```python
from build123d import *

# Parameters (mm, degrees)
EXTRUDE_1_DEPTH     = 3
SKETCH_2_R          = 2
SKETCH_2_W          = 80
SKETCH_2_H          = 35.5
CUT_EXTRUDE_1_DEPTH = 10
SKETCH_5_R          = 3
CUT_EXTRUDE_4_DEPTH = 234.518735865
FILLET_1_R          = 10
FILLET_2_R          = 3
FILLET_3_R          = 2


with BuildPart() as part:
    # 草图1 → 凸台-拉伸1 (new body)
    with BuildSketch(Plane(origin=(0, 0, 0), x_dir=(1, 0, 0), z_dir=(0, 1, 0))):
        with BuildLine():
            Line((-55, 0), (55, 0))
            Line((55, 0), (55, 35.5))
            Line((55, 35.5), (147.5, 35.5))
            Line((147.5, 35.5), (147.5, 66))
            Line((147.5, 66), (204, 66))
            Line((204, 66), (204, 26))
            Line((204, 26), (219, 26))
            Line((219, 26), (219, 73))
            ThreePointArc((219, 73), (216.656854249, 78.656854249), (211, 81))
            Line((211, 81), (132.5, 81))
            Line((132.5, 81), (132.5, 50.5))
            Line((132.5, 50.5), (-132.5, 50.5))
            Line((-132.5, 50.5), (-132.5, 81))
            Line((-132.5, 81), (-211, 81))
            ThreePointArc((-211, 81), (-216.656854249, 78.656854249), (-219, 73))
            Line((-219, 73), (-219, 26))
            Line((-219, 26), (-204, 26))
            Line((-204, 26), (-204, 66))
            Line((-204, 66), (-147.5, 66))
            Line((-147.5, 66), (-147.5, 35.5))
            Line((-147.5, 35.5), (-55, 35.5))
            Line((-55, 35.5), (-55, 0))
        make_face()
    extrude(amount=EXTRUDE_1_DEPTH)

    # 草图2 → 切除-拉伸1 (cut)
    with BuildSketch(Plane(origin=(0, 3, 0), x_dir=(1, 0, 0), z_dir=(0, 1, 0))):
        with Locations(Location((-47.5, 32.5, 0), (0, 0, 270))):
            Circle(SKETCH_2_R)
        with Locations(Location((-211.5, 33.5, 0), (0, 0, 270))):
            Circle(SKETCH_2_R)
        with Locations(Location((-211.5, 48.5, 0), (0, 0, 270))):
            Circle(SKETCH_2_R)
        with Locations(Location((211.5, 48.5, 0), (0, 0, 270))):
            Circle(SKETCH_2_R)
        with Locations(Location((211.5, 33.5, 0), (0, 0, 270))):
            Circle(SKETCH_2_R)
        with Locations(Location((-171.5, 73.5, 0), (0, 0, 270))):
            Circle(SKETCH_2_R)
        with Locations(Location((171.5, 73.5, 0), (0, 0, 270))):
            Circle(SKETCH_2_R)
        with Locations(Location((47.5, 32.5, 0), (0, 0, 270))):
            Circle(SKETCH_2_R)
        with Locations(Location((-47.5, 7.5, 0), (0, 0, 270))):
            Circle(SKETCH_2_R)
        with Locations(Location((-62.5, 43, 0), (0, 0, 270))):
            Circle(SKETCH_2_R)
        with Locations(Location((-126.999999701, 44.500000154, 0), (0, 0, 270))):
            Circle(SKETCH_2_R)
        with Locations(Location((62.5, 43, 0), (0, 0, 270))):
            Circle(SKETCH_2_R)
        with Locations(Location((126.999999701, 44.500000154, 0), (0, 0, 270))):
            Circle(SKETCH_2_R)
        with Locations(Location((47.5, 7.5, 0), (0, 0, 270))):
            Circle(SKETCH_2_R)
        with Locations((0, 17.75)):
            Rectangle(SKETCH_2_W, SKETCH_2_H)
    extrude(amount=-CUT_EXTRUDE_1_DEPTH, mode=Mode.SUBTRACT)

    # 草图5 → 切除-拉伸4 (cut, through all)
    with BuildSketch(Plane(origin=(0, 3, 0), x_dir=(1, 0, 0), z_dir=(0, 1, 0))):
        with Locations(Location((-211, 73, 0), (0, 0, 270))):
            Circle(SKETCH_5_R)
        with Locations(Location((211, 73, 0), (0, 0, 90))):
            Circle(SKETCH_5_R)
    extrude(amount=-CUT_EXTRUDE_4_DEPTH, mode=Mode.SUBTRACT)

    # 圆角1
    fillet_1_edges = [part.edges().sort_by_distance(p)[0] for p in [
        (-147.5, 1.5, -35.5),
        (-132.5, 1.5, -81),
        (132.5, 1.5, -81),
        (147.5, 1.5, -35.5),
    ]]
    fillet(fillet_1_edges, radius=FILLET_1_R)

    # 圆角2
    fillet_2_edges = [part.edges().sort_by_distance(p)[0] for p in [
        (55, 1.5, 0),
        (-55, 1.5, 0),
        (-55, 1.5, -35.5),
        (-204, 1.5, -66),
        (204, 1.5, -66),
        (55, 1.5, -35.5),
        (-40, 1.5, 0),
        (-40, 1.5, -35.5),
        (40, 1.5, -35.5),
        (40, 1.5, 0),
    ]]
    fillet(fillet_2_edges, radius=FILLET_2_R)

    # 圆角3
    fillet_3_edges = [part.edges().sort_by_distance(p)[0] for p in [
        (-147.5, 1.5, -66),
        (-204, 1.5, -26),
        (-219, 1.5, -26),
        (-132.5, 1.5, -50.5),
        (132.5, 1.5, -50.5),
        (219, 1.5, -26),
        (204, 1.5, -26),
        (147.5, 1.5, -66),
    ]]
    fillet(fillet_3_edges, radius=FILLET_3_R)


solid = part.part
```
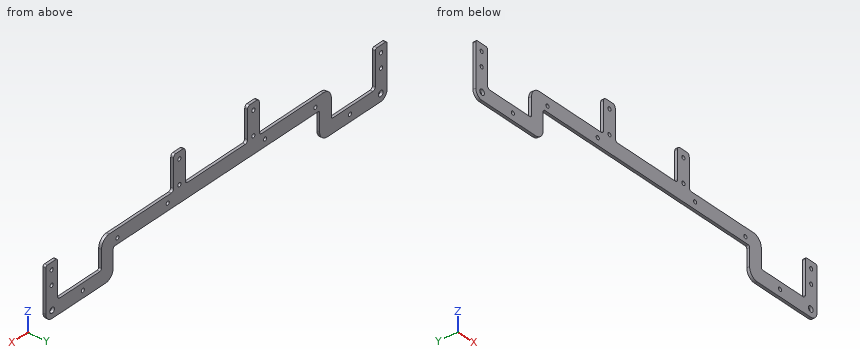
Verification items for the finished model (mm, model axes). Round coordinates to 2 decimals unless told otherwise and drop trailing zeros. Write each loop counter-clockwise with the first axis right and the second up, starting at its lowest first coordinate (ties: lowest second). Pieces come first, ordered by that corner, then holes.
1. Section check A-A on z = -15.5. Enter the section's corners in (x, y).
2. Scan lines: L1, parallel to X at y = 0.3, z = -28; L2, parallel to X at y = 1.85, z = -7; L3, parallel to X at y = 1.75, z = -14.5. Record each from-to range of solid material in increasing order.
3. Gauge pin test, flat ends, axial feed: P1, Ø1.5, axis at y = 1, z = -24.5, coming from the +X side; P2, Ø1.5, axis at x = -179, y = 1.5, coming from the +Z side; P3, Ø0.9, axis at x = -6.5, y = 1.5, coming from the +Z side. Record the tip position at first contact, or that the pin passes through.
4. Section check B-B on y = 1.6. State how many separate pieces and enclosed holes the cut face has, plus the area to 3 significant figures.
5. Section check C-C on x = 101. Enter the section's corners in (y, z).
Answer:
1. outline: (-55, 0) - (-40, 0) - (-40, 3) - (-55, 3) - close; (40, 0) - (55, 0) - (55, 3) - (40, 3) - close
2. L1: x = -219 to -204, -55 to -40, 40 to 55, 204 to 219
2. L2: x = -55 to -49.44, -45.56 to -40, 40 to 45.56, 49.44 to 55
2. L3: x = -55 to -40, 40 to 55
3. P1: stops at x = 55
3. P2: stops at z = -66
3. P3: stops at z = -35.5
4. separate pieces: 1
4. enclosed holes: 16
4. area: 9,410 mm2
5. outline: (0, -50.5) - (3, -50.5) - (3, -35.5) - (0, -35.5) - close
